Geometry: final body of the model. Coordinates: model frame, mm. Round coordinates to 2 decimals unless told otherwise and drop trailing zeros. Loops run counter-clockwise (first coordinate to the right, second up) from the corner with the lowest first, then second, coordinate; pieces in that order, holes last. Notation, with made-up numbers: M -12,-39.5 L 2,-39.5 A22 cw 2,-21.5 Z; hole C 25,-36.75 d1. An arc over 180 degrees is marked long. Answer as a JSON object with one key per item and string values.
Autodesk Inventor part; units mm, degrees
ref_plane "Start Plane" through (0, 0, 0) normal (1, 0, 0) x (0, 1, 0)
ref_plane "XZ Plane" through (0, 0, 0) normal (0, 1, 0) x (-1, 0, 0)
ref_plane "XY Plane" through (0, 0, 0) normal (0, 0, 1) x (1, 0, 0)
sketch "Main Sketch" plane through (0, 0, 0) normal (0, 0, 1) x (1, 0, 0)
  line L0 (0, 0) -> (109.7534, 0)
  line L1 (0, 0) -> (0, 9.525)
  line L2 (109.7534, 9.525) -> (109.7534, 0)
  line L3 (0, 9.525) -> (109.7534, 9.525)
  dimension "d3" = 19.05
revolve "Revolution1" add sketch "Main Sketch" angle 360 about axis through (0, 0, 0) along (1, 0, 0)
chamfer "Chamfer1" distance 2.54 angle 45 1 edges at (0, -9.525, 0) measured on face at (73.1689, 9.4941, -0.7664)
fillet "Fillet1" radius 2.54 1 edges at (109.7534, -9.525, 0)
properties part number "Shaft" material "Steel"
1) First-contact query: pin 1 (5 mm diameter, centred on y = 6, z = 7.5, fed in from +X); pin 2 (2 mm diameter, centred on x = 16.5, y = -1.5, fed in from +Z); pin 3 (6 mm diameter, centred on x = 54.5, y = 7.5, fed in from +Z) (3 decimals). Flat tips, straight axial feed; report the tip coordinate or a pass-through.
Geometry results:
{"pin 1": "x = 109.75", "pin 2": "z = 9.51", "pin 3": "z = 8.395"}
2) Cut plane A-A on x = 86.5. Return the cut outline in (y, z) (3 decimals).
Geometry results:
{"outline": "C 0,0 d19.05"}
3) Line query: probe 1 along Z at (x, y) = (95.5, 0) (3 decimals); probe 2 along Z at (x, y) = (32.5, 2); probe 3 along Y at (x, z) = (97, -5.25). Output: solid intervals per line, ascending.
Geometry results:
{"probe 1": "-9.525 to 9.525", "probe 2": "-9.31 to 9.31", "probe 3": "-7.95 to 7.95"}
